from build123d import *

# Parameters (mm, degrees)
F0_W     = 800
F0_H     = 1800
F1_DEPTH = 400
F2_W     = 180
F2_H     = 160
F3_DEPTH = 250
F2_W_2   = 80
F2_H_2   = 15
F4_DEPTH = 50
F5_R     = 7
F2_R     = 5
F6_DEPTH = 10
F7_W     = 150
F7_H     = 300
F8_DEPTH = 160


with BuildPart() as f1:
    # F0 (on Top) → F1 (new body)
    with BuildSketch(Plane.XY):
        Rectangle(F0_W, F0_H)
    extrude(amount=F1_DEPTH)

    # F2 (on face) → F3 (cut)
    with BuildSketch(Plane.XY.offset(400)):
        Polygon((0, 720), (0, 880), (-180, 880), (-180, 720), (-130, 720), (-80, 720), align=None)
        with Locations((90, 800)):
            Rectangle(F2_W, F2_H)
    extrude(amount=-F3_DEPTH, mode=Mode.SUBTRACT)

    # F2 (on face) → F4 (join)
    with BuildSketch(Plane.XY.offset(400)):
        Polygon((0, 880), (0, 895), (-195, 895), (-195, 705), (-130, 705), (-130, 720), (-180, 720), (-180, 880), align=None)
        Polygon((195, 895), (0, 895), (0, 880), (180, 880), (180, 720), (0, 720), (0, 705), (195, 705), align=None)
        with Locations((-40, 712.5)):
            Rectangle(F2_W_2, F2_H_2)
    extrude(amount=F4_DEPTH)

    # F5
    f5_edges = [f1.edges().sort_by_distance(p)[0] for p in [
        (0, 895, 450),
        (-195, 800, 450),
        (-162.5, 705, 450),
        (-130, 712.5, 450),
        (-155, 720, 450),
        (-180, 800, 450),
        (0, 880, 450),
        (180, 800, 450),
        (50, 720, 450),
        (-80, 712.5, 450),
        (57.5, 705, 450),
        (195, 800, 450),
        (-130, 705, 425),
        (-130, 720, 425),
        (-195, 705, 425),
        (195, 705, 425),
        (195, 895, 425),
        (-195, 895, 425),
    ]]
    fillet(f5_edges, radius=F5_R)

    # F2 (on face) → F6 (join)
    with BuildSketch(Plane.XY.offset(400)):
        with Locations((-300, 800)):
            Circle(F2_R)
        with Locations((300, 800)):
            Circle(F2_R)
    extrude(amount=F6_DEPTH)

    # F7 (on face) → F8 (cut)
    with BuildSketch(Plane.XZ.offset(900)):
        with Locations((275, 200)):
            Rectangle(F7_W, F7_H)
    extrude(amount=-F8_DEPTH, mode=Mode.SUBTRACT)


solid = f1.part
Model file for the job. Use its own axes, mm. A direction names the side the tool comes from. Round coordinates to 2 decimals unless told otherwise and drop trailing zeros. Loops run counter-clockwise (first coordinate to the right, second up) from the corner with the lowest first, then second, coordinate; pieces in that order, holes last.
1. Band-saw the part on C-C, the plane y = 98. List the corners of the cut face in (x, z).
Check values:
outline: (-400, 0) - (400, 0) - (400, 400) - (-400, 400) - close
2. Band-saw the part on A-A, the plane z = 319.5. List the corners of the cut face in (x, y).
Check values:
outline: (-400, -900) - (200, -900) - (200, -740) - (350, -740) - (350, -900) - (400, -900) - (400, 900) - (-400, 900) - close; hole (-180, 720) - (180, 720) - (180, 880) - (-180, 880) - close
3. Band-saw the part on D-D, the plane x = 4.5. List the corners of the cut face in (y, z), and give its area (3 significant figures).
Check values:
outline: (-900, 0) - (900, 0) - (900, 400) - (895, 400) - (895, 443) arc R7 ccw to (888, 450) - (887, 450) arc R7 ccw to (880, 443) - (880, 150) - (720, 150) - (720, 443) arc R7 ccw to (713, 450) - (712, 450) arc R7 ccw to (705, 443) - (705, 400) - (-900, 400) - close
area: 681,000 mm2
4. Mould opens along Y. For faces 1 (the flat face through (-400, -13, 197)), 2 (the flat face through (-6, 900, 197)), 3 (the flat face through (-3, 720, 299)) say: +Y half, -Y half, draft (parallel to the pull), parting line (faces both ways), or undercut.
Check values:
face 1: draft
face 2: +Y half
face 3: undercut
5. Drop flat-ended pins along their axis: P1, Ø21.5, axis at y = 761, z = 415, coming from the +X side; P2, Ø21.5, axis at x = 78, z = 423, coming from the +Y side; P3, Ø8, axis at x = -299.5, y = 801, coming from the +Z side. Give the stop position or say it passes through.
Check values:
P1: stops at x = 195
P2: stops at y = 895
P3: stops at z = 410
6. Band-saw the part on B-B, the plane x = 272. List the corners of the cut face in (y, z), and give its area (3 significant figures).
Check values:
outline: (-900, 0) - (900, 0) - (900, 400) - (-900, 400) - (-900, 350) - (-740, 350) - (-740, 50) - (-900, 50) - close
area: 672,000 mm2
7. Wall check: probe 1 along Y at (x, z) = (177, 274); probe 2 along Y at (x, z) = (56, 412.5); probe 3 along Z at (x, y) = (215.5, -589). Give the ranges that are in metal, low to high.
Check values:
probe 1: y = -900 to 720, 880 to 900
probe 2: y = 705 to 720, 880 to 895
probe 3: z = 0 to 400
8. Tool access for faces 4 (the flat face through (180, 801, 294)), 5 (the flat face through (200, -821, 198)), 6 (the flat face through (52, 705, 421)), 7 (the flat face through (3, 895, 421)): list every direction of +Z, -Z, +X, -X, +Y, -Y with a clear straight run to the whole face (end or side of a thin tool).
Check values:
face 4: +Z
face 5: -Y
face 6: +Z, +X, -X, -Y
face 7: +Z, +X, -X, +Y
